Geometry check sheet. Reference: drawing and pictorial views, mm from the part's lowest x, y, z. A direction names the side the tool comes from. Round coordinates to 2 decimals unless told otherwise and drop trailing zeros. Order: outer loops, then holes, each group sorted by start corner. A loop starts at its lowest first (then second) coordinate and runs counter-clockwise, first axis right, second up.
(1) Draft check along X on the marked faces 1, 2 and 3. Enter one of: pulls with the +X half, pulls with the -X half, needs draft (parallel to the pull), parting line crosses it, or undercut.
(2) Cross-section at A-A on y = 4. Count the separate pieces of the cut face and the enclosed holes in it, and give its area (3 significant figures).
(3) Set-up check for the marked faces 4, 5 and 6: record each of +Z, -Z, +X, -X, +Y, -Y from which the full face is reachable in a straight line by a thin tool's end or side.
(4) Cross-section at D-D on z = 33. Enter the section's corners in (x, y).
(5) Gauge pin test, flat ends, axial feed: P1, Ø1.9, axis at x = 89.5, y = 2, coming from the +Z side; P2, Ø3, axis at x = 3.5, y = 3, coming from the -Z side; P3, Ø3, axis at y = 2, z = 4.5, coming from the +X side; P4, Ø1, axis at x = 61.12, z = 36.83, coming from the +Y side. Record the tip position at first contact, or that the pin passes through.
(6) Thickness scan on L1, parallel to X at y = 3.2, z = 36.83; L2, parallel to Z at x = 13.5, y = 2.75 (1 decimal); L3, parallel to Z at x = 15.5, y = 5.5 (1 decimal). Record the ranges inside material, lowest first.
(7) Cross-section at C-C on z = 58.5. Enter the section's corners in (x, y).
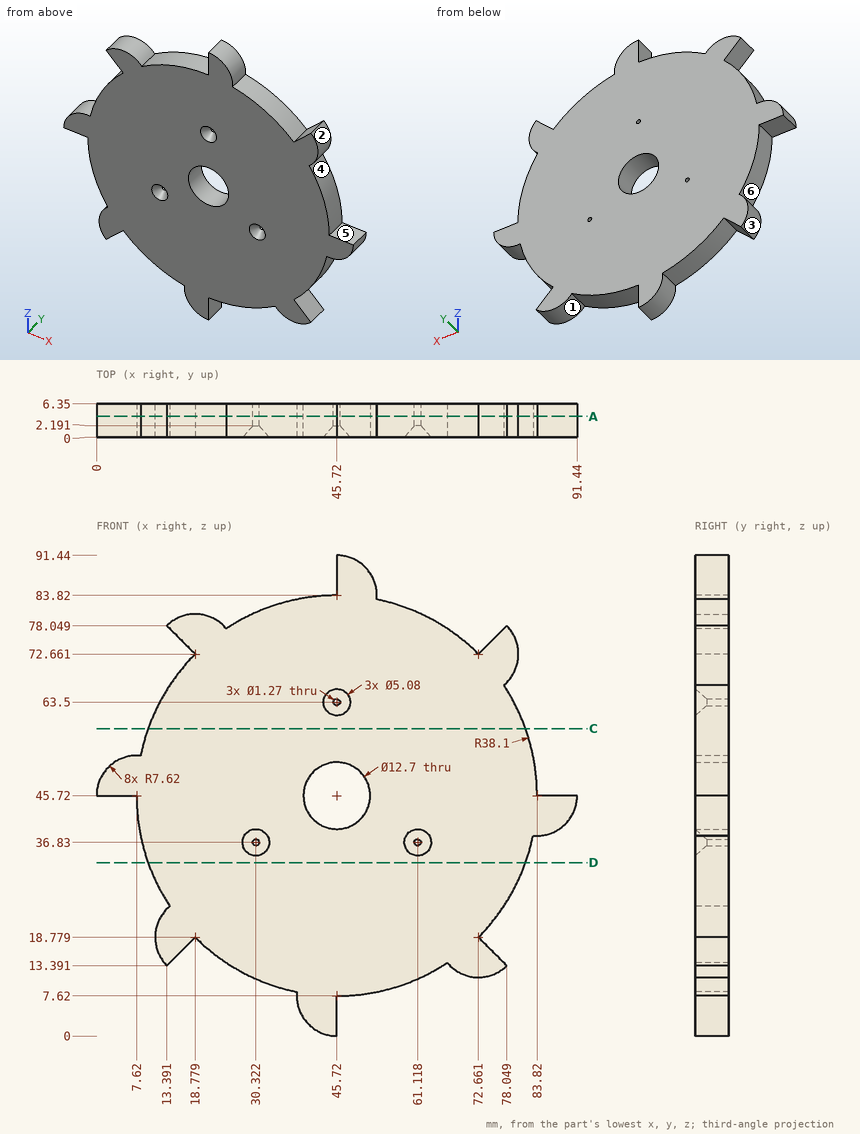
Found:
1. face 1: undercut
1. face 2: pulls with the +X half
1. face 3: pulls with the -X half
2. separate pieces: 1
2. enclosed holes: 4
2. area: 4,810 mm2
3. face 4: +X, +Y, -Y
3. face 5: +Z, +X, +Y, -Y
3. face 6: -X, +Y, -Y
4. outline: (9.81, 0) - (81.63, 0) - (81.63, 6.35) - (9.81, 6.35) - close
5. P1: stops at z = 45.72
5. P2: stops at z = 45.72
5. P3: stops at x = 45.72
5. P4: passes through
6. L1: x = 8.67 to 29.69, 30.96 to 60.48, 61.75 to 82.77
6. L2: z = 13.5 to 24.3, 25.4 to 66.1, 77.9 to 78.2
6. L3: z = 15.5 to 68.9, 75.9 to 79.5
7. outline: (9.83, 0) - (81.61, 0) - (81.61, 6.35) - (9.83, 6.35) - close
